Autodesk Inventor part; units mm, degrees
ref_plane "YZ Plane" through (0, 0, 0) normal (1, 0, 0) x (0, 1, 0)
ref_plane "XZ Plane" through (0, 0, 0) normal (0, 1, 0) x (-1, 0, 0)
ref_plane "XY Plane" through (0, 0, 0) normal (0, 0, 1) x (1, 0, 0)
sketch "Sketch1" plane through (0, 0, 0) normal (0, 0, 1) x (1, 0, 0)
  line L0 (-12.7, -25.4) -> (12.7, -25.4)
  line L1 (12.7, -25.4) -> (12.7, 25.4)
  line L2 (12.7, 25.4) -> (-12.7, 25.4)
  line L3 (-12.7, 25.4) -> (-12.7, -25.4)
  line L4 (-12.7, -25.4) -> (12.7, 25.4) construction
  line L5 (12.7, -25.4) -> (-12.7, 25.4) construction
  line L6 (-10.16, -22.86) -> (10.16, -22.86)
  line L7 (10.16, -22.86) -> (10.16, 22.86)
  line L8 (10.16, 22.86) -> (-10.16, 22.86)
  line L9 (-10.16, 22.86) -> (-10.16, -22.86)
  line L10 (-10.16, -22.86) -> (10.16, 22.86) construction
  line L11 (10.16, -22.86) -> (-10.16, 22.86) construction
  point P0 (0, 0)
  dimension "d0" = 25.4
  dimension "d1" = 50.8
  dimension "d2" = 20.32
  dimension "d3" = 45.72
extrude "Extrusion1" add sketch "Sketch1" along normal mid plane 368.3
sketch "Sketch2" plane through (-12.7, 25.4, 184.15) normal (0, 1, 0) x (1, 0, 0)
  line L0 (0, 368.3) -> (0, 0)
  line L1 (25.4, 0) -> (0, 0)
  point P0 (12.7, 184.15)
  point P1 (12.7, 6.35)
  dimension "d6" = 12.7
  dimension "d7" = 6.35
hole "Hole1" at (0, 25.4, 177.8) direction (0, -1, 0) diameter 4.1402 end through all
pattern_linear "Rectangular Pattern1" count 15 spacing 25.4 along (0, 0, -1) of "Hole1"
properties part number "Horizontal_frame_2nd_stage" material "Aluminum 6061"
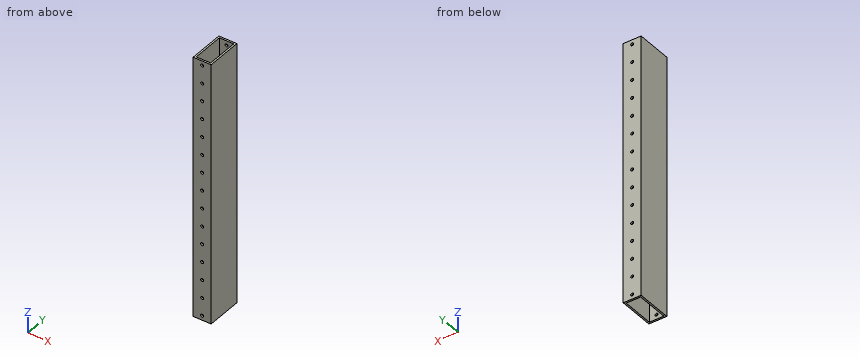
Could you check a few things on this model? Use its own coordinates, in mm. Coordinates: 2 decimals unless noted, no trailing zeros. Order: outer loops, then holes, each group sorted by start corner. A loop starts at its lowest first (then second) coordinate and runs counter-clockwise, first axis right, second up.
Q1. Please list where these lines run through material, in increasing order: L1, parallel to X at y = 3, z = -46.5; L2, parallel to Y at x = 7.75, z = 80.5; L3, parallel to X at y = -24.05, z = -177.8.
Q2. Suppose I cut it at A-A on x = 6.5. Please give me the cut outline in (y, z).
Q3. Suppose I cut it at C-C on y = -15. Please give me the cut outline in (x, z).
Q4. Suppose I cut it at B-B on z = -89. Please give me the cut outline in (x, y), and give its area (3 significant figures).
Q5. Will this pin go through, and if not, where does the flat tip stop? pin 1 (3.5 mm diameter, centred on x = 0, z = -127, fed in from +Y).
Answer:
1. L1: x = -12.7 to -10.16, 10.16 to 12.7
1. L2: y = -25.4 to -22.86, 22.86 to 25.4
1. L3: x = -12.7 to -2.07, 2.07 to 12.7
2. outline: (-25.4, -184.15) - (-22.86, -184.15) - (-22.86, 184.15) - (-25.4, 184.15) - close; (22.86, -184.15) - (25.4, -184.15) - (25.4, 184.15) - (22.86, 184.15) - close
3. outline: (-12.7, -184.15) - (-10.16, -184.15) - (-10.16, 184.15) - (-12.7, 184.15) - close; (10.16, -184.15) - (12.7, -184.15) - (12.7, 184.15) - (10.16, 184.15) - close
4. outline: (-12.7, -25.4) - (12.7, -25.4) - (12.7, 25.4) - (-12.7, 25.4) - close; hole (-10.16, -22.86) - (10.16, -22.86) - (10.16, 22.86) - (-10.16, 22.86) - close
4. area: 361 mm2
5. pin 1: passes through
